Autodesk Inventor part; units mm, degrees
ref_plane "YZ Plane" through (0, 0, 0) normal (1, 0, 0) x (0, 1, 0)
ref_plane "XZ Plane" through (0, 0, 0) normal (0, 1, 0) x (-1, 0, 0)
ref_plane "XY Plane" through (0, 0, 0) normal (0, 0, 1) x (1, 0, 0)
sketch "Sketch1" plane through (0, 0, 0) normal (0, 0, 1) x (1, 0, 0)
  line L0 (0, 0) -> (57.15, 0)
  line L1 (57.15, 0) -> (57.15, 50.8)
  line L2 (0, 50.8) -> (0, 0)
  line L3 (53.975, 50.8) -> (53.975, 3.175)
  line L4 (53.975, 3.175) -> (3.175, 3.175)
  line L5 (3.175, 3.175) -> (3.175, 50.8)
  line L6 (0, 50.8) -> (3.175, 50.8)
  line L7 (53.975, 50.8) -> (57.15, 50.8)
  dimension "d0" = 50.8
  dimension "d1" = 57.15
  dimension "d2" = 3.175
  dimension "d3" = 3.175
  dimension "d4" = 3.175
extrude "Extrusion1" add sketch "Sketch1" along normal blind 50.8
sketch "Sketch2" plane through (57.15, 0, 0) normal (1, 0, 0) x (0, 0, -1)
  line L0 (-50.8, 50.8) -> (-50.8, 0)
  line L1 (0, 0) -> (0, 50.8)
  line L2 (0, 50.8) -> (-50.8, 50.8)
  line L3 (0, 3.175) -> (-50.8, 3.175)
  circle A0 centre (-25.4, 31.75) radius 14.2875
  arc A1 (-6.749, 35.6286) -> (-44.051, 35.6286) centre (-25.4, 31.75) ccw
  line L4 (-44.051, 35.6286) -> (-50.8, 3.175)
  line L5 (-6.749, 35.6286) -> (0, 3.175)
  dimension "d7" = 28.575
  dimension "d8" = 25.4
  dimension "d9" = 19.05
extrude "Extrusion2" cut sketch "Sketch2" against normal through all contours L2 A1 L4 L0 | L2 L1 L5 A1 | A0
sketch "Sketch3" plane through (3.175, 3.175, 50.8) normal (0, 1, 0) x (1, 0, 0)
  line L0 (0, 0) -> (50.8, 0)
  line L1 (50.8, 50.8) -> (50.8, 0)
  line L2 (50.8, 50.8) -> (0, 50.8)
  circle A0 centre (25.4, 38.1) radius 3.175
  circle A1 centre (25.4, 12.7) radius 3.175
  line L3 (0, 50.8) -> (0, 0)
  point P0 (-3.175, 50.8)
  dimension "d12" = 6.35
  dimension "d13" = 6.35
  dimension "d14" = 12.7
  dimension "d15" = 25.4
  dimension "d16" = 12.7
  dimension "d17" = 25.4
  dimension "d20" = 50.8
extrude "Extrusion3" cut sketch "Sketch3" against normal blind 50.8 contours A0 | A1
equation "\"d3\" = d2"
equation "\"d4\" = d2"
equation "\"d12\" = d13"
equation "\"d15\" = 0.5 * d20"
equation "\"d16\" = d14"
equation "\"d17\" = d15"
properties part number "shooter bearing bracket"
Model file for the job. Use its own axes, mm. A direction names the side the tool comes from. Give positions to 0.01 mm unless a question says otherwise; leave off trailing zeros. Loops run counter-clockwise (first coordinate to the right, second up) from the corner with the lowest first, then second, coordinate; pieces in that order, holes last.
1) Saw through at A-A (z = 25.4). Count the separate pieces of the cut face and the enclosed holes in it, plus the area to 3 significant figures.
2) Tool access for faces 5 (the cylindrical face through (1.61, 50.797, 25.036)), 6 (the flat face through (53.975, 17, 25)): list every direction of +Z, -Z, +X, -X, +Y, -Y with a clear straight run to the whole face (end or side of a thin tool).
3) Pull direction X, two halves, no side cores. Call faces 1 (the flat face through (29, 3.175, 25)), 2 (the flat face through (57.15, 14, 25)), 3 (the flat face through (28, 0, 25)), 4 (the flat face through (0, 14, 25)): +X half, -X half, draft (parallel to the pull), parting line (faces both ways), or undercut.
4) Saw through at B-B (y = 45). Write the cut outline in (x, z) (3 decimals), plus the area to 3 significant figures.
5) Wall check: line 1 (X direction, y = 2, z = 12.7); line 2 (X direction, y = 7, z = 24) (3 decimals); line 3 (Y direction, x = 8.5, z = 21.5) (3 decimals). Give the ranges that are in metal, low to high.
6) Flat gauge pins, fed straight in: pin 1 Ø5.5 at (x, z) = (28.575, 38.1) entering from +Y; pin 2 Ø1.5 at (x, z) = (10, 30) entering from +Y (3 decimals). Where does each tip first touch, or does it go through?
7) Saw through at C-C (z = 38.1). Write the cut outline in (x, y) (3 decimals).
8) Saw through at D-D (y = 16). Write the cut outline in (x, z) (3 decimals), plus the area to 3 significant figures.
Answer block:
1. separate pieces: 3
1. enclosed holes: 0
1. area: 302 mm2
2. face 5: +X, -X, +Y
2. face 6: +Z, -Z, +Y
3. face 1: undercut
3. face 2: +X half
3. face 3: draft
3. face 4: -X half
4. outline: (0, 11.713) - (3.175, 11.713) - (3.175, 20.055) - (0, 20.055) - close; (0, 30.745) - (3.175, 30.745) - (3.175, 39.087) - (0, 39.087) - close; (53.975, 11.713) - (57.15, 11.713) - (57.15, 20.055) - (53.975, 20.055) - close; (53.975, 30.745) - (57.15, 30.745) - (57.15, 39.087) - (53.975, 39.087) - close
4. area: 106 mm2
5. line 1: x = 0 to 25.4, 31.75 to 57.15
5. line 2: x = 0 to 3.175, 53.975 to 57.15
5. line 3: y = 0 to 3.175
6. pin 1: passes through
6. pin 2: stops at y = 3.175
7. outline: (0, 0) - (25.4, 0) - (25.4, 3.175) - (3.175, 3.175) - (3.175, 25.205) - (0, 25.205) - close; (0, 38.295) - (3.175, 38.295) - (3.175, 45.949) - (0, 45.949) - close; (31.75, 0) - (57.15, 0) - (57.15, 25.205) - (53.975, 25.205) - (53.975, 3.175) - (31.75, 3.175) - close; (53.975, 38.295) - (57.15, 38.295) - (57.15, 45.949) - (53.975, 45.949) - close
8. outline: (0, 2.667) - (3.175, 2.667) - (3.175, 48.133) - (0, 48.133) - close; (53.975, 2.667) - (57.15, 2.667) - (57.15, 48.133) - (53.975, 48.133) - close
8. area: 289 mm2
